Work out the finished part from the listing and answer in its coordinate system (mm). Coordinates: 2 decimals unless noted, no trailing zeros. Answer as a JSON object with one key per item and string values. Group by question number.
1) Each of these flat-tipped pins is pushed along its axis until it touches: P1, Ø3, axis at x = -3, y = 7, coming from the -Z side; P2, Ø2.5, axis at y = 2.5, z = -55, coming from the -X side; P3, Ø5, axis at x = -10, y = 5.5, coming from the -Z side; P4, Ø4, axis at x = -7.5, z = -85.5, coming from the -Y side. Where does it stop, or does it pass through?
2) Find the intervals of material crossed by line 1 along X through (y, z) = (6.75, 17); line 2 along X through (y, z) = (3.75, -105); line 3 along X through (y, z) = (3.25, -35), in increasing order.
3) Section A-A (y = 2) is taken. Count the separate pieces of the cut face and the enclosed holes in it, plus the area to 3 significant figures.
from build123d import *

# Parameters (mm, degrees)
SKETCH1_W           = 34.833395016
SKETCH1_H           = 8
SKETCH1_W_2         = 5
SKETCH1_H_2         = 10
BOSS_EXTRUDE1_DEPTH = 10
FILLET1_R           = 10


with BuildPart() as part:
    # Sketch1 → Boss-Extrude1 (new body)
    with BuildSketch(Plane(origin=(0, 0, 0), x_dir=(1, 0, 0), z_dir=(0, 1, 0))):
        with BuildLine():
            Line((-34.833395016, 0), (0, 0))
            Line((0, 0), (0, 2))
            Line((0, 2), (-34.825702595, 2))
            ThreePointArc((-34.825702595, 2), (-34.831471904, 1.000007397), (-34.833395016, 0))
        make_face()
        Polygon((0, 2), (0, 0), (5, 0), (5, 130), (0, 130), (0, 122), (0, 120), (0, 112), (0, 110), (0, 102), (0, 100), (0, 92), (0, 90), (0, 82), (0, 80), (0, 72), (0, 70), (0, 62), (0, 60), (0, 52), (0, 50), (0, 42), (0, 40), (0, 32), (0, 30), (0, 22), (0, 20), (0, 12), (0, 10), align=None)
        with BuildLine():
            Line((-34.641016151, 10), (0, 10))
            Line((0, 10), (0, 12))
            Line((0, 12), (-34.556324308, 12))
            ThreePointArc((-34.556324308, 12), (-34.600595037, 11.000081508), (-34.641016151, 10))
        make_face()
        with BuildLine():
            Line((-39.833395016, 0), (-34.833395016, 0))
            ThreePointArc((-34.833395016, 0), (-34.831471904, 1.000007397), (-34.825702595, 2))
            ThreePointArc((-34.825702595, 2), (-34.764138624, 6.000710564), (-34.641016151, 10))
            ThreePointArc((-34.641016151, 10), (-34.600595037, 11.000081508), (-34.556324308, 12))
            ThreePointArc((-34.556324308, 12), (-34.340503133, 16.001901029), (-34.063022952, 20))
            ThreePointArc((-34.063022952, 20), (-33.98391775, 21.000156347), (-33.900953772, 22))
            ThreePointArc((-33.900953772, 22), (-33.529816222, 26.003108568), (-33.096826419, 30))
            ThreePointArc((-33.096826419, 30), (-32.978675002, 31.000232599), (-32.856649782, 32))
            ThreePointArc((-32.856649782, 32), (-32.328418622, 36.004344436), (-31.738046589, 40))
            ThreePointArc((-31.738046589, 40), (-31.580302492, 41.000310991), (-31.418663494, 42))
            ThreePointArc((-31.418663494, 42), (-30.730801915, 46.005620768), (-29.98041146, 50))
            ThreePointArc((-29.98041146, 50), (-29.782331047, 51.000392318), (-29.580328265, 52))
            ThreePointArc((-29.580328265, 52), (-28.729478957, 56.006950993), (-27.81560783, 60))
            ThreePointArc((-27.81560783, 60), (-27.576232201, 61.000477471), (-27.332899966, 62))
            ThreePointArc((-27.332899966, 62), (-26.314801256, 66.008350348), (-25.233075527, 70))
            ThreePointArc((-25.233075527, 70), (-24.951206094, 71.000567472), (-24.66533853, 72))
            ThreePointArc((-24.66533853, 72), (-23.474712485, 76.009836516), (-22.219732553, 80))
            ThreePointArc((-22.219732553, 80), (-21.893898758, 81.00066352), (-21.564017355, 82))
            ThreePointArc((-21.564017355, 82), (-20.194422544, 86.011430464), (-18.759613369, 90))
            ThreePointArc((-18.759613369, 90), (-18.388030357, 91.000767051), (-18.012341473, 92))
            ThreePointArc((-18.012341473, 92), (-16.455980001, 96.013157563), (-14.833395016, 100))
            ThreePointArc((-14.833395016, 100), (-14.413908154, 101.00087982), (-13.990247312, 102))
            ThreePointArc((-13.990247312, 102), (-12.237711236, 106.01504912), (-10.417774804, 110))
            ThreePointArc((-10.417774804, 110), (-9.947786552, 111.001004016), (-9.473545033, 112))
            ThreePointArc((-9.473545033, 112), (-7.513480483, 116.017144539), (-5.484646909, 120))
            ThreePointArc((-5.484646909, 120), (-4.961019464, 121.001142415), (-4.433046584, 122))
            ThreePointArc((-4.433046584, 122), (-2.25170348, 126.019494426), (0, 130))
            Line((0, 130), (-1.200062972, 134.853848871))
            ThreePointArc((-1.200062972, 134.853848871), (-3.00514583, 133.996135451), (-4.330127019, 132.5))
            ThreePointArc((-4.330127019, 132.5), (-30.803738983, 68.587046952), (-39.833395016, 0))
        make_face()
        with BuildLine():
            Line((-34.063022952, 20), (0, 20))
            Line((0, 20), (0, 22))
            Line((0, 22), (-33.900953772, 22))
            ThreePointArc((-33.900953772, 22), (-33.98391775, 21.000156347), (-34.063022952, 20))
        make_face()
        with BuildLine():
            Line((-33.096826419, 30), (0, 30))
            Line((0, 30), (0, 32))
            Line((0, 32), (-32.856649782, 32))
            ThreePointArc((-32.856649782, 32), (-32.978675002, 31.000232599), (-33.096826419, 30))
        make_face()
        with BuildLine():
            Line((-31.738046589, 40), (0, 40))
            Line((0, 40), (0, 42))
            Line((0, 42), (-31.418663494, 42))
            ThreePointArc((-31.418663494, 42), (-31.580302492, 41.000310991), (-31.738046589, 40))
        make_face()
        with BuildLine():
            Line((-29.98041146, 50), (0, 50))
            Line((0, 50), (0, 52))
            Line((0, 52), (-29.580328265, 52))
            ThreePointArc((-29.580328265, 52), (-29.782331047, 51.000392318), (-29.98041146, 50))
        make_face()
        with BuildLine():
            Line((-1.200062972, 134.853848871), (0, 130))
            Line((0, 130), (2.583616786, 134.280762117))
            ThreePointArc((2.583616786, 134.280762117), (0.748773929, 134.943615843), (-1.200062972, 134.853848871))
        make_face()
        with BuildLine():
            Line((0, 130), (5, 130))
            ThreePointArc((5, 130), (4.3541982, 132.457836047), (2.583616786, 134.280762117))
            Line((2.583616786, 134.280762117), (0, 130))
        make_face()
        with BuildLine():
            Line((0, 120), (0, 122))
            Line((0, 122), (-4.433046584, 122))
            ThreePointArc((-4.433046584, 122), (-4.961019464, 121.001142415), (-5.484646909, 120))
            Line((-5.484646909, 120), (0, 120))
        make_face()
        with BuildLine():
            Line((0, 110), (0, 112))
            Line((0, 112), (-9.473545033, 112))
            ThreePointArc((-9.473545033, 112), (-9.947786552, 111.001004016), (-10.417774804, 110))
            Line((-10.417774804, 110), (0, 110))
        make_face()
        with BuildLine():
            Line((0, 100), (0, 102))
            Line((0, 102), (-13.990247312, 102))
            ThreePointArc((-13.990247312, 102), (-14.413908154, 101.00087982), (-14.833395016, 100))
            Line((-14.833395016, 100), (0, 100))
        make_face()
        with BuildLine():
            Line((0, 90), (0, 92))
            Line((0, 92), (-18.012341473, 92))
            ThreePointArc((-18.012341473, 92), (-18.388030357, 91.000767051), (-18.759613369, 90))
            Line((-18.759613369, 90), (0, 90))
        make_face()
        with BuildLine():
            Line((0, 80), (0, 82))
            Line((0, 82), (-21.564017355, 82))
            ThreePointArc((-21.564017355, 82), (-21.893898758, 81.00066352), (-22.219732553, 80))
            Line((-22.219732553, 80), (0, 80))
        make_face()
        with BuildLine():
            Line((-25.233075527, 70), (0, 70))
            Line((0, 70), (0, 72))
            Line((0, 72), (-24.66533853, 72))
            ThreePointArc((-24.66533853, 72), (-24.951206094, 71.000567472), (-25.233075527, 70))
        make_face()
        with BuildLine():
            Line((-27.81560783, 60), (0, 60))
            Line((0, 60), (0, 62))
            Line((0, 62), (-27.332899966, 62))
            ThreePointArc((-27.332899966, 62), (-27.576232201, 61.000477471), (-27.81560783, 60))
        make_face()
        with Locations((-17.416697508, -4)):
            Rectangle(SKETCH1_W, SKETCH1_H)
        Polygon((-34.833395016, -8), (-34.833395016, 0), (-39.833395016, 0), (-39.833395016, -18), (-34.833395016, -18), align=None)
        with Locations((-37.333395016, -23)):
            Rectangle(SKETCH1_W_2, SKETCH1_H_2)
        with BuildLine():
            Line((0, -28), (0, -18))
            Line((0, -18), (-2.375046262, -18))
            ThreePointArc((-2.375046262, -18), (-4.875046262, -20.5), (-7.375046262, -18))
            Line((-7.375046262, -18), (-19.916697508, -18))
            Line((-19.916697508, -18), (-27.375046262, -18))
            ThreePointArc((-27.375046262, -18), (-29.875046262, -20.5), (-32.375046262, -18))
            Line((-32.375046262, -18), (-34.833395016, -18))
            Line((-34.833395016, -18), (-34.833395016, -28))
            Line((-34.833395016, -28), (0, -28))
        make_face()
        with BuildLine():
            Line((0, -18), (0, -8))
            Line((0, -8), (-34.833395016, -8))
            Line((-34.833395016, -8), (-34.833395016, -18))
            Line((-34.833395016, -18), (-32.375046262, -18))
            ThreePointArc((-32.375046262, -18), (-31.642813215, -16.232233047), (-29.875046262, -15.5))
            Line((-29.875046262, -15.5), (-4.875046262, -15.5))
            ThreePointArc((-4.875046262, -15.5), (-3.107279309, -16.232233047), (-2.375046262, -18))
            Line((-2.375046262, -18), (0, -18))
        make_face()
        with BuildLine():
            Line((-19.916697508, -18), (-7.375046262, -18))
            ThreePointArc((-7.375046262, -18), (-6.642813215, -16.232233047), (-4.875046262, -15.5))
            Line((-4.875046262, -15.5), (-29.875046262, -15.5))
            ThreePointArc((-29.875046262, -15.5), (-28.107279309, -16.232233047), (-27.375046262, -18))
            Line((-27.375046262, -18), (-19.916697508, -18))
        make_face()
        Polygon((5, 0), (0, 0), (0, -8), (0, -18), (0, -28), (5, -28), align=None)
    extrude(amount=BOSS_EXTRUDE1_DEPTH)

    # Fillet1
    fillet1_edges = [part.edges().sort_by_distance(p)[0] for p in [
        (5, 5, 28),
        (-39.833395016, 5, 28),
    ]]
    fillet(fillet1_edges, radius=FILLET1_R)


solid = part.part
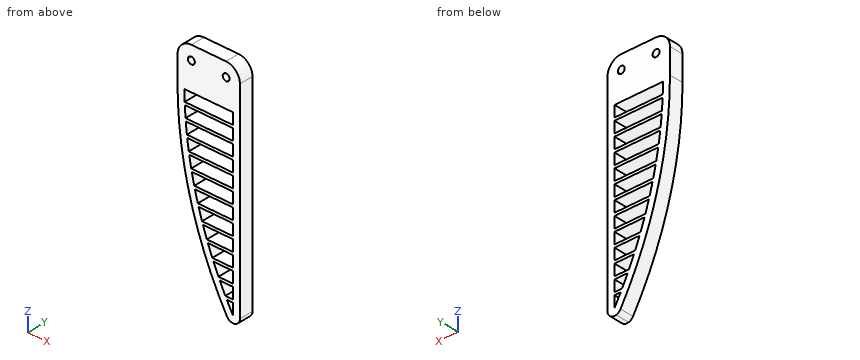
Report:
{
 "1": {"P1": "stops at z = -134.77", "P2": "stops at x = -34.33", "P3": "stops at z = -126.85", "P4": "passes through"},
 "2": {"line 1": "x = -39.83 to -32.17, -27.58 to -7.17, -2.58 to 5", "line 2": "x = -18.14 to -12.69, 0 to 5", "line 3": "x = -37.51 to -32.47, 0 to 5"},
 "3": {"separate pieces": "1", "enclosed holes": "15", "area": "3,180 mm²"}
}
